from build123d import *

# Parameters (mm, degrees)
F0_W     = 10.31875
F0_H     = 84.1375
F1_DEPTH = 1.5875
F2_W     = 19.05
F2_H     = 91.44
F3_DEPTH = 25.4
F4_W     = 10.31875
F4_H     = 84.1375
F5_DEPTH = 4.7625
F6_W     = 4.365625
F6_H     = 91.44
F7_DEPTH = 25.4


with BuildPart() as f1:
    # F0 (on Front) → F1 (new body)
    with BuildSketch(Plane.XZ):
        with Locations((-56.7394390884, 32.2464529891)):
            Rectangle(F0_W, F0_H)
    extrude(amount=F1_DEPTH)

    # F2 (on face) → F3 (join)
    with BuildSketch(Plane(origin=(0, 0, 0), x_dir=(-1, 0, 0), z_dir=(0, 1, 0))):
        with Locations((56.7394390884, 32.2464529891)):
            Rectangle(F2_W, F2_H)
    extrude(amount=F3_DEPTH)

    # F4 (on face) → F5 (cut)
    with BuildSketch(Plane.XZ.offset(1.5875)):
        with Locations((-56.7394390884, 32.2464529891)):
            Rectangle(F4_W, F4_H)
    extrude(amount=-F5_DEPTH, mode=Mode.SUBTRACT)

    # F6 (on face) → F7 (join)
    with BuildSketch(Plane.XZ):
        with Locations((-49.3972515884, 32.2464529891)):
            Rectangle(F6_W, F6_H)
    extrude(amount=F7_DEPTH)


solid = f1.part
Read the model definition and answer for the solid it produces. Units are mm, in the model's axes. A direction names the side the tool comes from. Give positions to 0.01 mm unless a question says otherwise; leave off trailing zeros. Write each loop counter-clockwise with the first axis right and the second up, starting at its lowest first coordinate (ties: lowest second). Pieces come first, ordered by that corner, then holes. Notation, with made-up numbers: M 45,-16 L 91,-16 A22 ccw 91,22 Z; hole C -15.75,57 d10. An arc over 180 degrees is marked long. One line per item, written item: value. Start each with the question number.
(1) Find section D-D (y = -21). Determine the outline of the cut face in (x, z), plus the area to 3 significant figures.
(2) Find section C-C (x = -61). Determine the outline of the cut face in (y, z) (3 decimals), plus the area to 3 significant figures.
(3) A tool of negligible diameter and unlimited length cuts with its end or side. For faces 1 (the flat face through (-63, 0, 32)), 2 (the flat face through (-57, 3.175, 33)), 3 (the flat face through (-49, -25.4, 33)), from which of +Z, -Z, +X, -X, +Y, -Y can it reach the whole face along a straight path? Write none if from no direction.
(4) Find section B-B (y = 2). Determine the outline of the cut face in (x, z), plus the area to 3 significant figures.
(5) Find the intervals of material crossed by line 1 (X direction, y = 2.5, z = 9.5); line 2 (Y direction, x = -59, z = 39) (3 decimals); line 3 (X direction, y = -11.5, z = 69), in increasing order.
(6) Flat-ended cylindrical pins translate along their axes: pin 1 Ø7.5 at (x, z) = (-55.5, 53) entering from -Y (3 decimals); pin 2 Ø4 at (x, y) = (-54, -12.5) entering from -Z; pin 3 Ø4 at (y, z) = (-16.5, 3) entering from -X; pin 4 Ø4 at (x, z) = (-63.5, 28) entering from -Y. Find the tip coordinate at first contact, or state that the pin passes through.
(7) Find section A-A (z = 3). Determine the outline of the cut face in (x, y) (3 decimals), plus the area to 3 significant figures.
(8) Determine the mould class of faces 4 (the flat face through (-55, 6, -13.474)), 5 (the flat face through (-66.264, 13, 32)), 6 (the flat face through (-61.899, 2, 32)) for opening direction X: pulls with the +X half, pulls with the -X half, needs draft (parallel to the pull), parting line crosses it, or undercut.
Results below:
1. outline: M -51.58,-13.47 L -47.21,-13.47 L -47.21,77.97 L -51.58,77.97 Z
1. area: 399 mm^2
2. outline: M 0,-13.474 L 25.4,-13.474 L 25.4,77.966 L 0,77.966 L 0,74.315 L 3.175,74.315 L 3.175,-9.822 L 0,-9.822 Z
2. area: 2,060 mm^2
3. face 1: +Z, -Z, -X, -Y
3. face 2: -Y
3. face 3: +Z, -Z, +X, -X, -Y
4. outline: M -66.26,-13.47 L -47.21,-13.47 L -47.21,77.97 L -66.26,77.97 Z; hole M -61.9,-9.82 L -51.58,-9.82 L -51.58,74.32 L -61.9,74.32 Z
4. area: 874 mm^2
5. line 1: x = -66.26 to -61.9, -51.58 to -47.21
5. line 2: y = 3.175 to 25.4
5. line 3: x = -51.58 to -47.21
6. pin 1: stops at y = 3.175
6. pin 2: passes through
6. pin 3: stops at x = -51.58
6. pin 4: stops at y = 0
7. outline: M -66.264,0 L -61.899,0 L -61.899,3.175 L -51.58,3.175 L -51.58,-25.4 L -47.214,-25.4 L -47.214,25.4 L -66.264,25.4 Z
7. area: 562 mm^2
8. face 4: needs draft
8. face 5: pulls with the -X half
8. face 6: undercut
